```python
from build123d import *

# Parameters (mm, degrees)
F0_W           = 914.4
F0_H           = 88.9
F1_DEPTH       = 19.05
F3_D           = 3.175
F3_DEPTH       = 12.7
F3_TIP         = 0.9538662327
F4_DEPTH       = 19.051
F6_D           = 3.175
F8_D           = 12.7
F8_CSINK_D     = 25.4
F8_CSINK_ANGLE = 90


with BuildPart() as f1:
    # F0 (on Front) → F1 (new body)
    with BuildSketch(Plane.XZ):
        with Locations((-107.1765102817, 24.4370475411)):
            Rectangle(F0_W, F0_H)
    extrude(amount=F1_DEPTH)

    # F3
    with Locations(Plane.XZ.offset(19.05)):
        with Locations((273.8234897183, 43.4870475411), (273.8234897183, 5.3870475411), (-488.1765102817, 43.4870475411), (-488.1765102817, 5.3870475411)):
            Hole(F3_D / 2, depth=F3_DEPTH)
            with Locations((0, 0, -(F3_DEPTH + F3_TIP / 2))):  # 118° drill point
                Cone(0, F3_D / 2, F3_TIP, mode=Mode.SUBTRACT)

    # F2 (on face) → F4 (cut, through all)
    with BuildSketch(Plane.XZ.offset(19.05)):
        with BuildLine():
            Line((197.6234897183, 37.1370475411), (197.6234897183, 68.8870475411))
            Line((197.6234897183, 68.8870475411), (184.9234897183, 68.8870475411))
            Line((184.9234897183, 68.8870475411), (184.9234897183, 49.8370475411))
            ThreePointArc((184.9234897183, 49.8370475411), (183.0636177789, 45.3469194806), (178.5734897183, 43.4870475411))
            Line((178.5734897183, 43.4870475411), (159.5234897183, 43.4870475411))
            ThreePointArc((159.5234897183, 43.4870475411), (164.0136177789, 41.6271756017), (165.8734897183, 37.1370475411))
            ThreePointArc((165.8734897183, 37.1370475411), (164.0136177789, 32.6469194806), (159.5234897183, 30.7870475411))
            Line((159.5234897183, 30.7870475411), (191.2734897183, 30.7870475411))
            ThreePointArc((191.2734897183, 30.7870475411), (195.7636177789, 32.6469194806), (197.6234897183, 37.1370475411))
        make_face()
    extrude(amount=-F4_DEPTH, mode=Mode.SUBTRACT)

    # F6 (through all)
    with Locations(Plane(origin=(0, 0, 0), x_dir=(-1, 0, 0), z_dir=(0, 1, 0))):
        with Locations((-324.6234897183, 11.7370475411), (538.9765102817, 11.7370475411)):
            Hole(F6_D / 2)

    # F8 (through all)
    with Locations(Plane(origin=(0, 0, 0), x_dir=(-1, 0, 0), z_dir=(0, 1, 0))):
        with Locations((-159.5234897183, 37.1370475411)):
            CounterSinkHole(F8_D / 2, F8_CSINK_D / 2, counter_sink_angle=F8_CSINK_ANGLE)


solid = f1.part
```
Here's how the part is built. I have some questions about the finished solid (model axes, mm). A direction names the side the tool comes from. Round coordinates to 2 decimals unless told otherwise and drop trailing zeros. Answer in a Markdown table with one row per item.
Item 1: Thinking about a two-plate mould opening in X: for faces 4 (the face through (169, -10, 43.487)), 5 (the face through (152.87, -6.04, 37.38)), 6 (the face through (-114, -9, -20.013)), 7 (the face through (-564.377, -9, 24)), which applies, +X half, -X half, draft (parallel to the pull), parting line (faces both ways), or undercut?
A:
| item | result |
|---|---|
| face 4 | undercut |
| face 5 | undercut |
| face 6 | draft |
| face 7 | -X half |
Item 2: For faces 1 (the face through (175, -10, 30.787)), 2 (the face through (184.923, -10, 59)), 3 (the face through (350.023, -9, 24)), which set-ups out of +Z, -Z, +X, -X, +Y, -Y let a thin tool reach every point of the face, with its end or its side?
A:
| item | result |
|---|---|
| face 1 | +Y, -Y |
| face 2 | +Z, +Y, -Y |
| face 3 | +Z, -Z, +X, +Y, -Y |
Item 3: If I drill on L1, parallel to X at y = -1.5, z = 55; L2, parallel to X at y = -14, z = 4; L3, parallel to X at y = -11, z = 37, over which ranges is the centre line in solid material (lowest first)? Write a range as from..to.
A:
| item | result |
|---|---|
| L1 | x = -564.38..184.92, 197.62..350.02 |
| L2 | x = -564.38..-488.95, -487.4..273.05, 274.6..350.02 |
| L3 | x = -564.38..153.17, 197.62..350.02 |
Item 4: I'm going to push flat-ended pins straight in: pin 1 (1.9 mm diameter, centred on x = 273.82, z = 43.49, fed in from -Y); pin 2 (2.5 mm diameter, centred on x = -488.18, z = 43.49, fed in from -Y). Where does each tip first touch, or does it pass through?
A:
| item | result |
|---|---|
| pin 1 | stops at y = -5.97 |
| pin 2 | stops at y = -6.15 |
